Geometry check sheet. Reference: the model listing, model coordinates, mm. Face numbers are marked on the shaded views. A direction names the side the tool comes from. Round coordinates to 2 decimals unless told otherwise and drop trailing zeros. Loops run counter-clockwise (first coordinate to the right, second up) from the corner with the lowest first, then second, coordinate; pieces in that order, holes last. Notation, with made-up numbers: M 51.25,11 L 83.25,11 A30 cw 83.25,46 Z; hole C 4.5,79.5 d9. An arc over 180 degrees is marked long. Use one line per item in the form item = value. Start each with the question number.
1. Cross-section at D-D (y = -3.5). Record the boundary of the cut face in (x, z).
2. Set-up check for the marked faces 1, 2, 3 and 4: record each of +Z, -Z, +X, -X, +Y, -Y from which the full face is reachable in a straight line by a thin tool's end or side.
3. Cross-section at C-C (x = -2.75). Record the boundary of the cut face in (y, z) (1 decimal).
4. Material ranges on line 1 (Z direction, x = 5.25, y = 3.25); line 2 (Z direction, x = 4.25, y = -1.5); line 3 (Z direction, x = -4.5, y = 0), recorded low to high.
5. Go/stop test with flat-tipped pins: pin 1 (5 mm diameter, centred on x = -4.5, y = -1, fed in from +Z); pin 2 (4 mm diameter, centred on x = -4.5, y = -1, fed in from +Z); pin 3 (5 mm diameter, centred on x = -0.5, y = -3.5, fed in from +Z). Record where each tip stops, or that it passes through.
6. Cross-section at A-A (y = 0). Record the boundary of the cut face in (x, z).
```python
from build123d import *

# Parameters (mm, degrees)
F0_W         = 9.525
F0_H         = 9.525
F1_DEPTH     = 2.286
F2_T1_DEPTH  = 21.3619144247
F3_W         = 2.9083
F3_H         = 9.525
F3_W_2       = 6.8834
F4_DEPTH     = 1.905
F5_R         = 1.6556676611
F6_W         = 12.7
F6_H         = 1.27
F7_DEPTH     = 4.191
F8_SIZE2     = 8.7232408068
F8_SIZE      = 3.175
F9_T4_DEPTH  = 12.7
F9_T9_DEPTH  = 12.7
F10_T1_DEPTH = 20.1155023365


# Not quite as in the source:
# - a fillet or chamfer that OpenCascade refuses, or shapes differently, is made with other operations: its cross-section is extruded or revolved along the edge and cut away or added


with BuildPart() as f1:
    # F0 (on Top) → F1 (new body)
    with BuildSketch(Plane.XY):
        Rectangle(F0_W, F0_H)
    extrude(amount=F1_DEPTH)

    # F2: chamfer of 1.3208 x 2.2876927066 on 2 edges, made by hand

    # F2_s2 → F2_t1 (cut)
    with BuildSketch(Plane.XZ.offset(-10.6809572123)):
        Polygon((-4.7625, -0.0016927066), (-3.4417, 2.286), (-4.7625, 2.286), align=None)
        Polygon((4.7625, -0.0016927066), (3.4417, 2.286), (4.7625, 2.286), align=None)
    extrude(amount=F2_T1_DEPTH, mode=Mode.SUBTRACT)

    # F3 (on face) → F4 (join)
    with BuildSketch(Plane.XY.offset(2.286)):
        with Locations((4.89585, 0)):
            Rectangle(F3_W, F3_H)
        Rectangle(F3_W_2, F3_H)
        with Locations((-4.89585, 0)):
            Rectangle(F3_W, F3_H)
    extrude(amount=F4_DEPTH)

    # F5
    f5_edges = [f1.edges().sort_by_distance(p)[0] for p in [
        (0, 4.7625, 4.191),
        (0, -4.7625, 4.191),
    ]]
    fillet(f5_edges, radius=F5_R)

    # F6 (on face) → F7 (join)
    with BuildSketch(Plane.XY.offset(4.191)):
        Rectangle(F6_W, F6_H)
    extrude(amount=F7_DEPTH)

    # F8
    f8_edges = [f1.edges().sort_by_distance(p)[0] for p in [
        (-6.35, 0, 8.382),
    ]]
    f8_side = f1.faces().sort_by_distance((-6.35, 0, 3.935532))[0]
    chamfer(f8_edges, length=F8_SIZE, length2=F8_SIZE2, reference=f8_side)

    # F9: fillet of radius 2.8207671263 on 2 edges, made by hand


with BuildPart() as f9_tool2:
    # F9_s3 → F9_t4 (new body)
    with BuildSketch(Plane.YZ.offset(-6.35)):
        with BuildLine():
            ThreePointArc((-0.635, 6.9981468006), (-1.3849039981, 5.0828783899), (-3.235890411, 4.1859623453))
            Line((-3.235890411, 4.1859623453), (-3.2139027394, 3.9047438998))
            ThreePointArc((-3.2139027394, 3.9047438998), (-3.1068323389, 3.9089232874), (-0.635, 3.9089232874))
            Line((-0.635, 3.9089232874), (-0.3529232874, 4.191))
            Line((-0.3529232874, 4.191), (-0.3529232874, 6.9981468006))
            Line((-0.3529232874, 6.9981468006), (-0.635, 6.9981468006))
        make_face()
    extrude(amount=F9_T4_DEPTH)

    split(bisect_by=Plane(origin=(-2.4163064349, 0, 6.6387473684), x_dir=(0, 1, 0), z_dir=(0.3420201433, 0, -0.9396926208)), keep=Keep.TOP)


with BuildPart() as f1_1:
    add(f1.part)

    # F9_t1: union F9_tool2
    add(f9_tool2.part)


with BuildPart() as f9_tool7:
    # F9_s8 → F9_t9 (new body)
    with BuildSketch(Plane.YZ.offset(6.35)):
        with BuildLine():
            ThreePointArc((0.635, 6.9981468006), (1.3849039981, 5.0828783899), (3.235890411, 4.1859623453))
            Line((3.235890411, 4.1859623453), (3.2139027394, 3.9047438998))
            ThreePointArc((3.2139027394, 3.9047438998), (3.1068323389, 3.9089232874), (0.635, 3.9089232874))
            Line((0.635, 3.9089232874), (0.3529232874, 4.191))
            Line((0.3529232874, 4.191), (0.3529232874, 6.9981468006))
            Line((0.3529232874, 6.9981468006), (0.635, 6.9981468006))
        make_face()
    extrude(amount=-F9_T9_DEPTH)

    split(bisect_by=Plane(origin=(-2.4163064349, 0, 6.6387473684), x_dir=(0, 1, 0), z_dir=(0.3420201433, 0, -0.9396926208)), keep=Keep.TOP)


with BuildPart() as f1_2:
    add(f1_1.part)

    # F9_t6: union F9_tool7
    add(f9_tool7.part)

    # F10: fillet of radius 5.08 on 1 edges, made by hand

    # F10_s2 → F10_t1 (cut)
    with BuildSketch(Plane.XZ.offset(-10.0577511683)):
        with BuildLine():
            ThreePointArc((-6.35, 2.286), (-5.2774477357, 4.8097508006), (-3.0493882968, 6.4083244148))
            Line((-3.0493882968, 6.4083244148), (-3.0841375434, 6.5037971851))
            Line((-3.0841375434, 6.5037971851), (-6.3847492466, 5.3024727703))
            Line((-6.3847492466, 5.3024727703), (-6.4516, 5.207))
            ThreePointArc((-6.4516, 5.207), (-6.4516, 3.7465), (-6.4507614806, 2.299026282))
            Line((-6.4507614806, 2.299026282), (-6.35, 2.286))
        make_face()
    extrude(amount=F10_T1_DEPTH, mode=Mode.SUBTRACT)


solid = f1_2.part
```
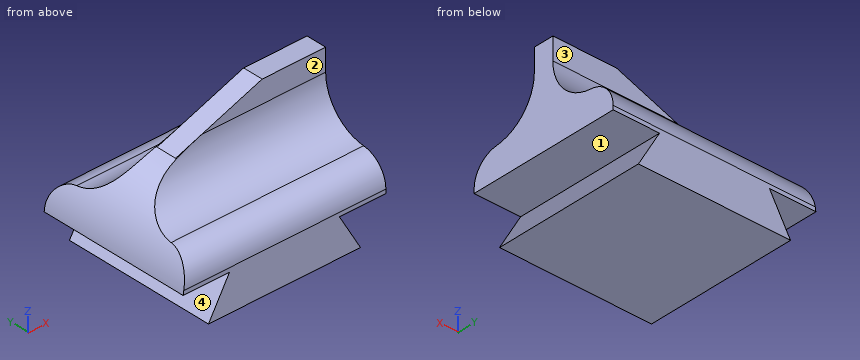
Reported:
q1.outline = M -6.35,2.29 L -3.44,2.29 L -4.76,0 L 4.76,0 L 3.44,2.29 L 6.35,2.29 L 6.35,4.14 L -5.73,4.14 A5.08 ccw Z
q2.face_1 = +X, +Y, -Y
q2.face_2 = +Z, +X, -X, -Y
q2.face_3 = +Z, +X, -X, +Y
q2.face_4 = -X, +Y, -Y
q3.outline = M -4.8,0 L 4.8,0 L 4.8,2.5 A1.7 ccw 3.2,4.2 A2.8 cw 0.7,6.5 L -0.7,6.5 A2.8 cw -3.2,4.2 A1.7 ccw -4.8,2.5 Z
q4.line_1 = 2.29 to 4.18
q4.line_2 = 0 to 0.89, 2.29 to 4.97
q4.line_3 = 0 to 0.45, 2.29 to 5.59
q5.pin_1 = 6.78
q5.pin_2 = 6.6
q5.pin_3 = 5.61
q6.outline = M -6.35,2.29 L -3.44,2.29 L -4.76,0 L 4.76,0 L 3.44,2.29 L 6.35,2.29 L 6.35,8.38 L 2.37,8.38 L -3.05,6.41 A5.08 ccw Z
